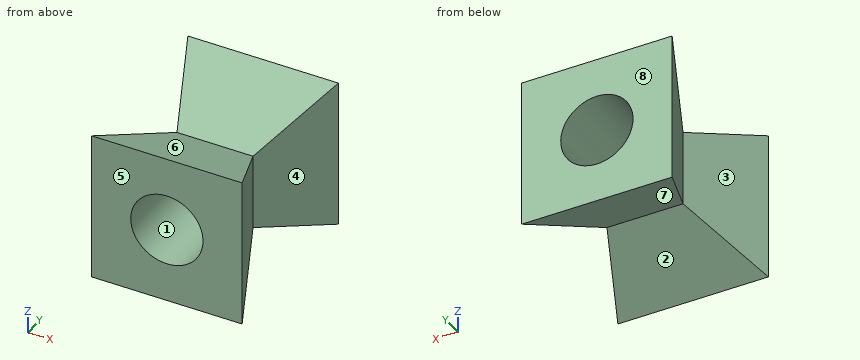
from build123d import *

# Parameters (mm, degrees)
SKETCH1_W           = 104
SKETCH1_H           = 121.112050925
BOSS_EXTRUDE1_DEPTH = 104
CUT_EXTRUDE1_DEPTH  = 104
CUT_EXTRUDE2_DEPTH  = 104
CUT_EXTRUDE3_DEPTH  = 191.525927053
CUT_EXTRUDE4_DEPTH  = 191.525927053
SKETCH6_R           = 25
CUT_EXTRUDE5_DEPTH  = 191.525927053


with BuildPart() as part:
    # Sketch1 → Boss-Extrude1 (new body)
    with BuildSketch(Plane.XY):
        with Locations((52, 60.556025463)):
            Rectangle(SKETCH1_W, SKETCH1_H)
    extrude(amount=BOSS_EXTRUDE1_DEPTH)

    # Sketch2 → Cut-Extrude1 (cut)
    with BuildSketch(Plane(origin=(0, 0, 0), x_dir=(-1, 0, 0), z_dir=(0, 0, -1))):
        Polygon((0, 121.112050925), (-25.704507779, 60.556025463), (0, 0), align=None)
    extrude(amount=-CUT_EXTRUDE1_DEPTH, mode=Mode.SUBTRACT)

    # Sketch3 → Cut-Extrude2 (cut)
    with BuildSketch(Plane(origin=(0, 0, 0), x_dir=(-1, 0, 0), z_dir=(0, 0, -1))):
        Polygon((-104, 121.112050925), (-78.295492221, 60.556025463), (-104, 0), align=None)
    extrude(amount=-CUT_EXTRUDE2_DEPTH, mode=Mode.SUBTRACT)

    # Sketch4 → Cut-Extrude3 (cut, through all)
    with BuildSketch(Plane(origin=(0, 0, 0), x_dir=(0, 0, -1), z_dir=(1, 0, 0))):
        Polygon((-104, 121.112050925), (-78.295492221, 60.556025463), (-104, 0), align=None)
    extrude(amount=CUT_EXTRUDE3_DEPTH, mode=Mode.SUBTRACT)

    # Sketch5 → Cut-Extrude4 (cut, through all)
    with BuildSketch(Plane(origin=(0, 0, 0), x_dir=(0, 0, -1), z_dir=(1, 0, 0))):
        Polygon((0, 121.112050925), (-25.704507779, 60.556025463), (0, 0), align=None)
    extrude(amount=CUT_EXTRUDE4_DEPTH, mode=Mode.SUBTRACT)

    # Sketch6 → Cut-Extrude5 (cut, through all)
    with BuildSketch(Plane(origin=(0, 121.112050925, 0), x_dir=(1, 0, 0), z_dir=(0, 1, 0))):
        with Locations(Location((52, -52, 0), (0, 0, 270))):
            Circle(SKETCH6_R)
    extrude(amount=-CUT_EXTRUDE5_DEPTH, mode=Mode.SUBTRACT)


solid = part.part
Work out the finished part from the listing and answer in its coordinate system (mm). Face numbers are marked on the shaded views. A direction names the side the tool comes from. Give positions to 0.01 mm unless a question says otherwise; leave off trailing zeros. Write each loop counter-clockwise with the first axis right and the second up, starting at its lowest first coordinate (ties: lowest second). Pieces come first, ordered by that corner, then holes. Notation, with made-up numbers: (8, 77.25) - (20, 77.25) arc R24 cw to (20, 90.25) - close; hole circle Ø10 at (62, 66.5). An arc over 180 degrees is marked (long way). One line per item, written item: value. Start each with the question number.
1. For a pull along Z with two mould halves and no side action, classify the marked faces 1, 2 and 3 as +Z half, -Z half, draft (parallel to the pull), parting line (faces both ways), or undercut.
2. Consider probe 1 along Z at (x, y) = (53, 72); probe 2 along X at (y, z) = (57, 52); probe 3 along X at (y, z) = (68, 52). Determine where each line is inside the solid, lowest interval first.
3. Find section D-D (y = 109). Write down the section's boundary in (x, z), then the cut area to 3 significant figures.
4. Find section C-C (x = 96). Write down the section's boundary in (y, z).
5. Find section A-A (z = 45). Write down the section's boundary in (x, y), then the cut area to 3 significant figures.
6. For the marked faces 4, 5, 6, 7 and 8, determine the directions among +Z, -Z, +X, -X, +Y, -Y from which every point of the face is accessible in a straight line to the end or side of a thin tool.
7. Given pin 1 (12 mm diameter, centred on x = 33.5, y = 106, fed in from -Z); pin 2 (5 mm diameter, centred on x = 22, y = 32.5, fed in from -Z); pin 3 (12 mm diameter, centred on y = 53.5, z = 77.5, fed in from +X), each flat-ended and moving along its own axis, determine where each tip first touches the part or whether it passes through.
8. Find section B-B (x = 52). Write down the section's boundary in (y, z), then the cut area to 3 significant figures.
Geometry results:
1. face 1: undercut
1. face 2: -Z half
1. face 3: draft
2. probe 1: 20.85 to 27.02, 76.98 to 83.15
2. probe 2: 24.2 to 27, 77 to 79.8
2. probe 3: 22.54 to 27, 77 to 81.46
3. outline: (5.14, 5.14) - (98.86, 5.14) - (98.86, 98.86) - (5.14, 98.86) - close; hole circle Ø50 at (52, 52)
3. area: 6,820 mm2
4. outline: (0, 0) - (18.85, 8) - (18.85, 96) - (0, 104) - close; (102.27, 8) - (121.11, 0) - (121.11, 104) - (102.27, 96) - close
5. outline: (0, 0) - (28, 0) - (28, 121.11) - (0, 121.11) - (25.7, 60.56) - close; (76, 0) - (104, 0) - (78.3, 60.56) - (104, 121.11) - (76, 121.11) - close
5. area: 3,670 mm2
6. face 4: +Z, -Z, +X
6. face 5: +Z, -Z, +X, -X, -Y
6. face 6: +Z, +X, -X
6. face 7: -Z, +X, -X
6. face 8: +Z, -Z, +X, -X, +Y
7. pin 1: z = 3.87
7. pin 2: z = 12.73
7. pin 3: x = 83.84
8. outline: (0, 0) - (60.56, 25.7) - (121.11, 0) - (121.11, 27) - (0, 27) - close; (0, 77) - (121.11, 77) - (121.11, 104) - (60.56, 78.3) - (0, 104) - close
8. area: 3,430 mm2
